```python
from build123d import *

# Parameters (mm, degrees)
CYLINDER_R     = 18
CYLINDER_DEPTH = 30


with BuildPart() as cilindro:
    # Cylinder → Cylinder (new body)
    with BuildSketch(Plane.XY.offset(-3)):
        Circle(CYLINDER_R)
    extrude(amount=CYLINDER_DEPTH)


with BuildPart() as cut:
    # Cone → Cone (revolve)
    with BuildSketch(Plane.XZ):
        Polygon((0, 0), (23.3, 0), (23, 25), (0, 25), align=None)
    revolve(axis=Axis((0, 0, 0), (0, 0, 1)))

    # Cut: cut Cilindro
    add(cilindro.part, mode=Mode.SUBTRACT)


solid = cut.part
```
The listing builds one solid part. Answer for the finished solid, in the listing's coordinates (mm). Round coordinates to 2 decimals unless told otherwise and drop trailing zeros. Write each loop counter-clockwise with the first axis right and the second up, starting at its lowest first coordinate (ties: lowest second). Pieces come first, ordered by that corner, then holes. Notation, with made-up numbers: (15.5, 25.5) -> (44.5, 25.5) arc R23 ccw to (44.5, 51.5) -> close; hole circle Ø9 at (26, 55). An arc over 180 degrees is marked (long way). Use CSV: the item, a comma, the result in double quotes. Start each with the question number.
(1) Section A-A on z = 8 is taken. Give the vertices of the cut face in (x, y).
(2) Each of these flat-tipped pins is pushed along its axis until it touches: pin 1 (6 mm diameter, centred on x = -14.5, z = 21.5, fed in from -Y); pin 2 (4 mm diameter, centred on y = -0.5, z = 19.5, fed in from +X); pin 3 (10 mm diameter, centred on x = -9.5, z = 16.5, fed in from -Y). Where does it stop, or does it pass through?
(3) Consider L1, parallel to X at y = -16, z = 2; L2, parallel to X at y = 0, z = 8; L3, parallel to Y at x = 0, z = 9.5. Determine where each line is inside the solid, lowest interval first. Write a range as from..to.
(4) The mould has two halves that part along X. Classify faces 1 (the face through (-18.369, -14.085, 12.675)), 2 (the face through (-2.343, 17.847, 12.325)), 3 (the face through (-12, -14, 0)): released by +X, released by -X, zero draft, split by the parting line, or undercut.
(5) Section B-B on z = 18.5 is taken. Give the vertices of the cut face in (x, y).
A:
1,outline,"circle Ø46.41 at (0, 0); hole circle Ø36 at (0, 0)"
2,pin 1,"stops at y = -19.97"
2,pin 2,"stops at x = 23.09"
2,pin 3,"stops at y = -22.66"
3,L1,"x = -16.9..-8.25, 8.25..16.9"
3,L2,"x = -23.2..-18, 18..23.2"
3,L3,"y = -23.19..-18, 18..23.19"
4,face 1,"split by the parting line"
4,face 2,"undercut"
4,face 3,"zero draft"
5,outline,"circle Ø46.16 at (0, 0); hole circle Ø36 at (0, 0)"
